Build history of the part. All positions in model axes, mm. A direction names the side the tool comes from. Round coordinates to 2 decimals unless told otherwise and drop trailing zeros. Write each loop counter-clockwise with the first axis right and the second up, starting at its lowest first coordinate (ties: lowest second). Pieces come first, ordered by that corner, then holes.
Item 1: Drop flat-ended pins along their axis: pin 1 Ø14.5 at (x, z) = (103.5, 6) entering from +Y; pin 2 Ø22 at (x, y) = (43.5, 14.5) entering from -Z; pin 3 Ø6 at (y, z) = (9.5, 2) entering from +X. Give the stop position or say it passes through.
Item 2: Band-saw the part on C-C, the plane y = -19. Write the cut outline in (x, z).
Item 3: Band-saw the part on A-A, the plane z = 8. Write the cut outline in (x, y).
Item 4: 3-axis set-ups, long thin cutter, end or side, ignore diameter. For faces 1 (the flat face through (6.14, 10.98, 20.14)), 2 (the flat face through (-18, 10, 20.348)), 3 (the flat face through (-4, 24.1, 10)), 4 (the flat face through (-24.62, -1.7, 10.32)): which of +Z, -Z, +X, -X, +Y, -Y reach the whole face in a straight line?
Item 5: Mould opens along Y. For faces 5 (the flat face through (107, 24, 10)), 6 (the flat face through (-34, -44.1, 7)), 7 (the cylindrical face through (112.073, 10.196, 8.699)), 8 (the flat face through (-31, 10, 0)) say: +Y half, -Y half, draft (parallel to the pull), parting line (faces both ways), or undercut.
Item 6: Wall check: probe 1 along X at (y, z) = (7, 10); probe 2 along X at (y, z) = (20.5, 7); probe 3 along Y at (x, z) = (89.5, 4). Give the ranges that are in metal, low to high.
Item 7: Band-saw the part on B-B, the plane x = -12.5. Write the cut outline in (y, z), then the cut area to 3 significant figures.
Item 8: Band-saw the part on D-D, the plane x = 50. Write the cut outline in (y, z), then the cut area to 3 significant figures.
```python
from build123d import *

# Parameters (mm, degrees)
BOSS_EXTRUDE3_START = -4
BOSS_EXTRUDE3_DEPTH = 28
SKETCH3_R           = 6
CUT_EXTRUDE1_DEPTH  = 28
BOSS_EXTRUDE4_START = 10
SKETCH5_W           = 77
SKETCH5_H           = 20
BOSS_EXTRUDE4_DEPTH = 10
BOSS_EXTRUDE5_DEPTH = 2
BOSS_EXTRUDE6_DEPTH = 54.1
CUT_EXTRUDE5_REACH  = 151.158
SKETCH9_W           = 9.998489886
SKETCH9_H           = 40


with BuildPart() as part:
    # Sketch1 → Boss-Extrude3 (new body)
    with BuildSketch(Plane(origin=(0, 0, 0), x_dir=(1, 0, 0), z_dir=(0, 1, 0)).offset(BOSS_EXTRUDE3_START)):
        with BuildLine():
            Line((117.93, 4.45), (82.93, 4.45))
            Line((82.93, 4.45), (82.93, -24.45))
            Line((82.93, -24.45), (117.93, -24.45))
            ThreePointArc((117.93, -24.45), (132.38, -10), (117.93, 4.45))
        make_face()
    extrude(amount=BOSS_EXTRUDE3_DEPTH)

    # Sketch3 → Cut-Extrude1 (cut)
    with BuildSketch(Plane(origin=(0, 24, 0), x_dir=(1, 0, 0), z_dir=(0, 1, 0))):
        with Locations(Location((117.93, -10, 0), (0, 0, 270))):
            Circle(SKETCH3_R)
    extrude(amount=-CUT_EXTRUDE1_DEPTH, mode=Mode.SUBTRACT)

    # Sketch5 → Boss-Extrude4 (add, symmetric)
    with BuildSketch(Plane(origin=(0, 0, 0), x_dir=(1, 0, 0), z_dir=(0, 1, 0)).offset(BOSS_EXTRUDE4_START)):
        with Locations((44.43, -10)):
            Rectangle(SKETCH5_W, SKETCH5_H)
    extrude(amount=BOSS_EXTRUDE4_DEPTH, both=True)

    # Sketch6 → Boss-Extrude5 (add)
    with BuildSketch(Plane.XY):
        Polygon((-39.16, 64.1), (-39.16, -44.1), (-9.24, -44.1), (-4.836934731, -41.448091963), (15.93, -4.1), (15.93, 24.1), (-4.836934731, 61.448091963), (-9.24, 64.1), align=None)
    extrude(amount=-BOSS_EXTRUDE5_DEPTH)

    # Sketch7 → Boss-Extrude6 (add, symmetric)
    with BuildSketch(Plane(origin=(0, 10, 0), x_dir=(-1, 0, 0), z_dir=(0, -1, 0))):
        Polygon((-15.93, 0), (-15.93, -10.35), (-5.931510114, -20.348489886), (26.278489886, -20.348489886), (39.16, -20.348489886), (39.16, 0), align=None)
    extrude(amount=BOSS_EXTRUDE6_DEPTH, both=True)

    # Cut-Extrude5: up to this face of the body (flat: up to its plane)
    cut_extrude5_end = Plane(part.part.faces().sort_by_distance((8.383659054, -30.874400728, 0))[0])
    # Sketch9 → Cut-Extrude5 (cut, up to the picked face)
    with BuildSketch(Plane.XY.offset(20.348489886), mode=Mode.PRIVATE) as cut_extrude5_sk1:
        with Locations((10.930755057, -24.1)):
            Rectangle(SKETCH9_W, SKETCH9_H)
    cut_extrude5_tool1 = split(extrude(cut_extrude5_sk1.sketch, amount=-CUT_EXTRUDE5_REACH, mode=Mode.PRIVATE), bisect_by=cut_extrude5_end, keep=Keep.BOTH, mode=Mode.PRIVATE)
    # Sketch9 → Cut-Extrude5 (cut, up to the picked face)
    with BuildSketch(Plane.XY.offset(20.348489886), mode=Mode.PRIVATE) as cut_extrude5_sk2:
        Polygon((5.931510114, -44.1), (5.931510114, -4.1), (-22.92, -4.1), (-33.526601718, -14.706601718), (-33.526601718, -44.1), align=None)
    cut_extrude5_tool2 = split(extrude(cut_extrude5_sk2.sketch, amount=-CUT_EXTRUDE5_REACH, mode=Mode.PRIVATE), bisect_by=cut_extrude5_end, keep=Keep.BOTH, mode=Mode.PRIVATE)
    # Sketch9 → Cut-Extrude5 (cut, up to the picked face)
    with BuildSketch(Plane.XY.offset(20.348489886), mode=Mode.PRIVATE) as cut_extrude5_sk3:
        with Locations((10.930755057, 44.1)):
            Rectangle(SKETCH9_W, SKETCH9_H)
    cut_extrude5_tool3 = split(extrude(cut_extrude5_sk3.sketch, amount=-CUT_EXTRUDE5_REACH, mode=Mode.PRIVATE), bisect_by=cut_extrude5_end, keep=Keep.BOTH, mode=Mode.PRIVATE)
    # Sketch9 → Cut-Extrude5 (cut, up to the picked face)
    with BuildSketch(Plane.XY.offset(20.348489886), mode=Mode.PRIVATE) as cut_extrude5_sk4:
        Polygon((-22.92, 24.1), (5.931510114, 24.1), (5.931510114, 64.1), (-33.526601718, 64.1), (-33.526601718, 34.706601718), align=None)
    cut_extrude5_tool4 = split(extrude(cut_extrude5_sk4.sketch, amount=-CUT_EXTRUDE5_REACH, mode=Mode.PRIVATE), bisect_by=cut_extrude5_end, keep=Keep.BOTH, mode=Mode.PRIVATE)
    # Sketch9 → Cut-Extrude5 (cut, up to the picked face)
    with BuildSketch(Plane.XY.offset(20.348489886), mode=Mode.PRIVATE) as cut_extrude5_sk5:
        Polygon((-22.92, 0), (-22.92, 20), (-26.278489886, 23.358489886), (-39.16, 23.358489886), (-39.16, -3.358489886), (-26.278489886, -3.358489886), align=None)
    cut_extrude5_tool5 = split(extrude(cut_extrude5_sk5.sketch, amount=-CUT_EXTRUDE5_REACH, mode=Mode.PRIVATE), bisect_by=cut_extrude5_end, keep=Keep.BOTH, mode=Mode.PRIVATE)
    add(cut_extrude5_tool1.solids().sort_by(Axis((10.930755, -24.1, 20.34849), (0, 0, -1)))[0], mode=Mode.SUBTRACT)
    add(cut_extrude5_tool2.solids().sort_by(Axis((-13.199096, -24.708463, 20.34849), (0, 0, -1)))[0], mode=Mode.SUBTRACT)
    add(cut_extrude5_tool3.solids().sort_by(Axis((10.930755, 44.1, 20.34849), (0, 0, -1)))[0], mode=Mode.SUBTRACT)
    add(cut_extrude5_tool4.solids().sort_by(Axis((-13.199096, 44.708463, 20.34849), (0, 0, -1)))[0], mode=Mode.SUBTRACT)
    add(cut_extrude5_tool5.solids().sort_by(Axis((-31.226846, 10, 20.34849), (0, 0, -1)))[0], mode=Mode.SUBTRACT)


solid = part.part
```
Results:
1. pin 1: stops at y = 24
1. pin 2: stops at z = 0
1. pin 3: stops at x = 131.49
2. outline: (-39.16, -2) - (7.65, -2) - (7.65, 0) - (-33.53, 0) - (-33.53, 20.35) - (-39.16, 20.35) - close
3. outline: (-39.16, -44.1) - (-33.53, -44.1) - (-33.53, -14.71) - (-22.92, -4.1) - (15.93, -4.1) - (15.93, 0) - (82.93, 0) - (82.93, -4) - (112.27, -4) - (112.27, 24) - (82.93, 24) - (82.93, 20) - (15.93, 20) - (15.93, 24.1) - (-22.92, 24.1) - (-33.53, 34.71) - (-33.53, 64.1) - (-39.16, 64.1) - (-39.16, 23.36) - (-26.28, 23.36) - (-22.92, 20) - (-22.92, 0) - (-26.28, -3.36) - (-39.16, -3.36) - close; (123.59, -4) - (132.24, -4) - (132.24, 24) - (123.59, 24) - close
4. face 1: +Z
4. face 2: +Z, -X, +Y, -Y
4. face 3: +Z, +X, +Y
4. face 4: +Z, -X
5. face 5: +Y half
5. face 6: -Y half
5. face 7: draft
5. face 8: undercut
6. probe 1: x = -22.92 to 111.93, 123.93 to 132.38
6. probe 2: x = -23.42 to 15.93, 82.93 to 112.73, 123.13 to 132.07
6. probe 3: y = -4 to 24
7. outline: (-44.1, -2) - (64.1, -2) - (64.1, 0) - (24.1, 0) - (24.1, 20.35) - (-4.1, 20.35) - (-4.1, 0) - (-44.1, 0) - close
7. area: 790 mm2
8. outline: (0, 0) - (20, 0) - (20, 20) - (0, 20) - close
8. area: 400 mm2
